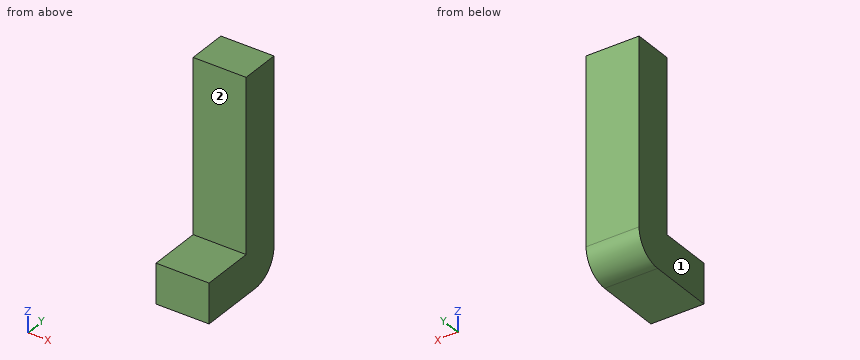
from build123d import *

# Parameters (mm, degrees)
F0_W     = 76.2
F0_H     = 330.2
F1_DEPTH = 101.6


# Not quite as in the source:
# - a feature of the source that left no trace in its solid (it failed there, or was rolled back) is left out


with BuildPart() as f1:
    # F0 (on Right) → F1 (new body)
    with BuildSketch(Plane.YZ):
        with Locations((-103.380974756, -25.9231243968)):
            Rectangle(F0_W, F0_H)
        with BuildLine():
            Line((-65.280974756, -191.0231243968), (-141.480974756, -191.0231243968))
            Line((-141.480974756, -191.0231243968), (-243.080974756, -191.0231243968))
            Line((-243.080974756, -191.0231243968), (-243.080974756, -267.2231243968))
            Line((-243.080974756, -267.2231243968), (-116.080974756, -267.2231243968))
            ThreePointArc((-116.080974756, -267.2231243968), (-80.1599502717, -252.3441488811), (-65.280974756, -216.4231243968))
            Line((-65.280974756, -216.4231243968), (-65.280974756, -191.0231243968))
        make_face()
    extrude(amount=F1_DEPTH)


solid = f1.part
Can you work these out from the model? Positions are in its coordinate system, mm. Face numbers are marked on the shaded views. A direction names the side the tool comes from. Coordinates: 2 decimals unless noted, no trailing zeros. Loops run counter-clockwise (first coordinate to the right, second up) from the corner with the lowest first, then second, coordinate; pieces in that order, holes last. Notation, with made-up numbers: M 82.5,59 L 131.5,59 A11 cw 131.5,63 Z; hole C -14.75,-20 d11. An arc over 180 degrees is marked long. Answer as CSV lines item,"result". Start each with the question number.
1. Suppose I cut it at B-B, the plane z = 78. List the corners of the cut face in (x, y) for me.
2. If I drill on probe 1 along Y at (x, z) = (83, 60); probe 2 along Z at (x, y) = (93.5, -217.5); probe 3 along Z at (x, y) = (23.5, -115.5), over which ranges is the centre line in solid material (lowest first)? Write a range as [from, to].
3. For pin 1 Ø1.5 at (x, z) = (88.5, 92) entering from -Y; pin 2 Ø1.5 at (x, y) = (21.5, -196) entering from +Z; pin 3 Ø6 at (x, z) = (84, -225) entering from +Y, each with a flat end and sliding along its axis, tell me the tip position at first contact or that it passes through.
4. Suppose I cut it at A-A, the plane x = 63. List the corners of the cut face in (y, z) for me.
5. Suppose I cut it at C-C, the plane y = -183.5. List the corners of the cut face in (x, z) for me, plus the area to 3 significant figures.
6. For the marked faces 1 and 2, which set-ups out of +Z, -Z, +X, -X, +Y, -Y let a thin tool reach every point of the face, with its end or its side?
Output:
1,outline,"M 0,-141.48 L 101.6,-141.48 L 101.6,-65.28 L 0,-65.28 Z"
2,probe 1,"y = [-141.48, -65.28]"
2,probe 2,"z = [-267.22, -191.02]"
2,probe 3,"z = [-267.22, 139.18]"
3,pin 1,"stops at y = -141.48"
3,pin 2,"stops at z = -191.02"
3,pin 3,"stops at y = -65.59"
4,outline,"M -243.08,-267.22 L -116.08,-267.22 A50.8 ccw -65.28,-216.42 L -65.28,139.18 L -141.48,139.18 L -141.48,-191.02 L -243.08,-191.02 Z"
5,outline,"M 0,-267.22 L 101.6,-267.22 L 101.6,-191.02 L 0,-191.02 Z"
5,area,"7,740 mm^2"
6,face 1,"+Z, -Z, -X, +Y, -Y"
6,face 2,"+Z, +X, -X, -Y"
